Source: CAD feature listing. Evaluate the final solid. Frame: model axes, mm. Face numbers are marked on the shaded views. A direction names the side the tool comes from. Give positions to 0.01 mm unless a question says otherwise; leave off trailing zeros. Order: outer loops, then holes, each group sorted by start corner. A loop starts at its lowest first (then second) coordinate and runs counter-clockwise, first axis right, second up.
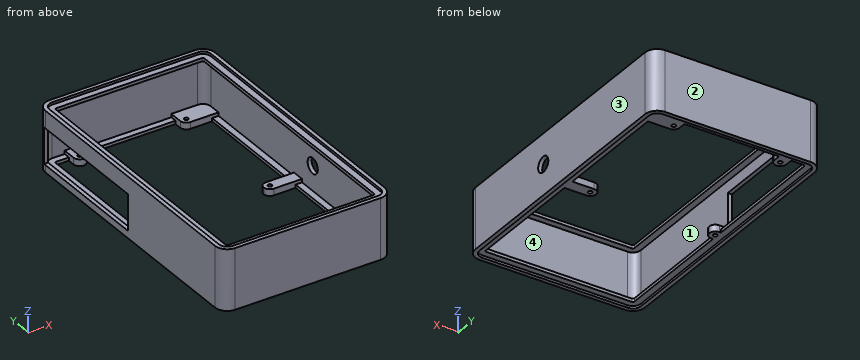
from build123d import *

# Parameters (mm, degrees)
SKETCH1_W               = 210
SKETCH1_H               = 350
SKETCH1_W_2             = 200
SKETCH1_H_2             = 340
BOSS_EXTRUDE1_DEPTH     = 75
FILLET1_R               = 15
FILLET2_R               = 10
BOSS_EXTRUDE2_START     = -4
BOSS_EXTRUDE2_DEPTH     = 4
CUT_EXTRUDE1_DEPTH      = 4
CUT_EXTRUDE1_DEPTH_BACK = 25
SKETCH3_W               = 44.5
SKETCH3_H               = 156.13
SKETCH3_H_2             = 2.62
SKETCH4_W               = 2
SKETCH4_H               = 2.62
CUT_EXTRUDE2_DEPTH      = 18
BOSS_EXTRUDE4_START     = -4
SKETCH5_R               = 2.55
BOSS_EXTRUDE4_DEPTH     = 8.23
SKETCH6_R               = 9.55
CUT_EXTRUDE4_DEPTH      = 22
CUT_EXTRUDE5_START      = -22
CUT_EXTRUDE5_DEPTH      = 22


with BuildPart() as part:
    # Sketch1 → Boss-Extrude1 (new body)
    with BuildSketch(Plane.XY):
        with Locations((105, 175)):
            Rectangle(SKETCH1_W, SKETCH1_H)
        with Locations((105, 175)):
            Rectangle(SKETCH1_W_2, SKETCH1_H_2, mode=Mode.SUBTRACT)
    extrude(amount=BOSS_EXTRUDE1_DEPTH)

    # Fillet1
    fillet1_edges = [part.edges().sort_by_distance(p)[0] for p in [
        (0, 350, 37.5),
        (210, 350, 37.5),
        (210, 0, 37.5),
        (0, 0, 37.5),
    ]]
    fillet(fillet1_edges, radius=FILLET1_R)

    # Fillet2
    fillet2_edges = [part.edges().sort_by_distance(p)[0] for p in [
        (5, 5, 37.5),
        (205, 5, 37.5),
        (205, 345, 37.5),
        (5, 345, 37.5),
    ]]
    fillet(fillet2_edges, radius=FILLET2_R)

    # Sketch2 → Boss-Extrude2 (add)
    with BuildSketch(Plane(origin=(0, 0, 3), x_dir=(-1, 0, 0), z_dir=(0, 0, -1)).offset(BOSS_EXTRUDE2_START)):
        with BuildLine():
            Line((-15, 5), (-195, 5))
            ThreePointArc((-195, 5), (-202.071067812, 7.928932188), (-205, 15))
            Line((-205, 15), (-205, 335))
            ThreePointArc((-205, 335), (-202.071067812, 342.071067812), (-195, 345))
            Line((-195, 345), (-15, 345))
            ThreePointArc((-15, 345), (-7.928932188, 342.071067812), (-5, 335))
            Line((-5, 335), (-5, 15))
            ThreePointArc((-5, 15), (-7.928932188, 7.928932188), (-15, 5))
        make_face()
        with BuildLine():
            Line((-13, 335), (-13, 15))
            ThreePointArc((-13, 15), (-13.585786438, 13.585786438), (-15, 13))
            Line((-15, 13), (-195, 13))
            ThreePointArc((-195, 13), (-196.414213562, 13.585786438), (-197, 15))
            Line((-197, 15), (-197, 335))
            ThreePointArc((-197, 335), (-196.414213562, 336.414213562), (-195, 337))
            Line((-195, 337), (-15, 337))
            ThreePointArc((-15, 337), (-13.585786438, 336.414213562), (-13, 335))
        make_face(mode=Mode.SUBTRACT)
    boss_extrude2 = extrude(amount=BOSS_EXTRUDE2_DEPTH)

    # Mirror1: Boss-Extrude2 across plane
    add(boss_extrude2.mirror(Plane(origin=(0, 0, 37.5), x_dir=(1, 0, 0), z_dir=(0, 0, -1))))

    # Sketch3 → Cut-Extrude1 (cut, two sides: drawn at the far end of the back side and taken through both)
    with BuildSketch(Plane(origin=(5, 0, 0), x_dir=(0, 0, -1), z_dir=(1, 0, 0)).offset(-CUT_EXTRUDE1_DEPTH_BACK)):
        with Locations((-31.25, 256.935)):
            Rectangle(SKETCH3_W, SKETCH3_H)
        with Locations((-31.25, 336.31)):
            Rectangle(SKETCH3_W, SKETCH3_H_2)
    extrude(amount=CUT_EXTRUDE1_DEPTH + CUT_EXTRUDE1_DEPTH_BACK, mode=Mode.SUBTRACT)

    # Sketch4 → Cut-Extrude2 (cut)
    with BuildSketch(Plane(origin=(5, 0, 0), x_dir=(0, 0, -1), z_dir=(1, 0, 0))):
        with Locations((-54.5, 336.31)):
            Rectangle(SKETCH4_W, SKETCH4_H)
        Polygon((-9, 337.62), (-53.5, 337.62), (-55.5, 337.62), (-55.5, 339.62), (-7, 339.62), (-7, 337.62), align=None)
        with Locations((-8, 336.31)):
            Rectangle(SKETCH4_W, SKETCH4_H)
    extrude(amount=CUT_EXTRUDE2_DEPTH, mode=Mode.SUBTRACT)

    # Sketch5 → Boss-Extrude4 (add)
    # profile 1 of 4: a face of its own
    with BuildSketch(Plane.XY.offset(7).offset(BOSS_EXTRUDE4_START)):
        with BuildLine():
            Line((15.06, 178.09), (5, 178.09))
            Line((5, 178.09), (5, 163.09))
            Line((5, 163.09), (15.06, 163.09))
            ThreePointArc((15.06, 163.09), (20.363300859, 165.286699141), (22.56, 170.59))
            ThreePointArc((22.56, 170.59), (20.363300859, 175.893300859), (15.06, 178.09))
        make_face()
        with Locations((15.06, 170.59)):
            Circle(SKETCH5_R, mode=Mode.SUBTRACT)
    # profile 2 of 4: a face of its own
    with BuildSketch(Plane.XY.offset(7).offset(BOSS_EXTRUDE4_START)):
        with BuildLine():
            Line((205, 163.09), (205, 178.09))
            Line((205, 178.09), (170, 178.09))
            ThreePointArc((170, 178.09), (164.696699141, 175.893300859), (162.5, 170.59))
            ThreePointArc((162.5, 170.59), (164.696699141, 165.286699141), (170, 163.09))
            Line((170, 163.09), (205, 163.09))
        make_face()
        with Locations((170, 170.59)):
            Circle(SKETCH5_R, mode=Mode.SUBTRACT)
    # profile 3 of 4: a face of its own
    with BuildSketch(Plane.XY.offset(7).offset(BOSS_EXTRUDE4_START)):
        with BuildLine():
            Line((195, 345), (162.5, 345))
            Line((162.5, 345), (162.5, 328.07))
            ThreePointArc((162.5, 328.07), (164.696699141, 322.766699141), (170, 320.57))
            Line((170, 320.57), (205, 320.57))
            Line((205, 320.57), (205, 335))
            ThreePointArc((205, 335), (202.071067812, 342.071067812), (195, 345))
        make_face()
        with Locations(Location((170, 328.07, 0), (0, 0, 180))):
            Circle(SKETCH5_R, mode=Mode.SUBTRACT)
    # profile 4 of 4: a face of its own
    with BuildSketch(Plane.XY.offset(7).offset(BOSS_EXTRUDE4_START)):
        with BuildLine():
            Line((45.42, 345), (30.42, 345))
            Line((30.42, 345), (30.42, 328.07))
            ThreePointArc((30.42, 328.07), (37.92, 320.57), (45.42, 328.07))
            Line((45.42, 328.07), (45.42, 345))
        make_face()
        with Locations((37.92, 328.07)):
            Circle(SKETCH5_R, mode=Mode.SUBTRACT)
    extrude(amount=BOSS_EXTRUDE4_DEPTH)

    # Sketch6 → Cut-Extrude4 (cut)
    with BuildSketch(Plane(origin=(210, 0, 0), x_dir=(0, 0, -1), z_dir=(1, 0, 0))):
        with Locations((-37.5, 143)):
            Circle(SKETCH6_R)
    extrude(amount=-CUT_EXTRUDE4_DEPTH, mode=Mode.SUBTRACT)

    # Sketch7 → Cut-Extrude5 (cut)
    with BuildSketch(Plane.XY.offset(11.23).offset(CUT_EXTRUDE5_START)):
        with BuildLine():
            Line((13, 169.087036261), (13, 172.092963739))
            ThreePointArc((13, 172.092963739), (12.51, 170.59), (13, 169.087036261))
        make_face()
    extrude(amount=CUT_EXTRUDE5_DEPTH, mode=Mode.SUBTRACT)


solid = part.part
(1) Section C-C, the plane y = 143. Return loops of the section in (x, z).
(2) Draft query along Z for the marked faces 1 and 2. Return one class per face: +Z half, -Z half, draft (parallel to the pull), parting line (faces both ways), or undercut.
(3) Section D-D, the plane x = 190.5. Return loops of the section in (y, z), plus the area to 3 significant figures.
(4) Line query: line 1 along X through (y, z) = (170.59, 6); line 2 along Y through (x, z) = (15.06, 5.5); line 3 along Y through (x, z) = (37.92, 7.25). Output: solid intervals per line, ascending.
(5) Section A-A, the plane y = 50.5. Return loops of the section in (x, z), plus the area to 3 significant figures.
(6) Section B-B, the plane x = 117. Return loops of the section in (y, z).
(7) Access query for the marked faces 3 and 4. Directions: +Z, -Z, +X, -X, +Y, -Y. A direction counts if a zero-diameter tool reaches every point of the face in a straight line with its end or side. Return the directions, or none.
(8) Pin query (flat end, axial travel): pin 1 Ø7.5 at (x, y) = (41, 329) entering from +Z; pin 2 Ø11.5 at (y, z) = (143, 37.5) entering from +X; pin 3 Ø1.4 at (x, z) = (3, 41.5) entering from -Y. Return the tip coordinate at first contact, or that it passes through.
Checks:
1. outline: (0, 0) - (5, 0) - (5, 3) - (13, 3) - (13, 7) - (5, 7) - (5, 68) - (13, 68) - (13, 72) - (5, 72) - (5, 75) - (0, 75) - close; (197, 3) - (205, 3) - (205, 0) - (210, 0) - (210, 27.95) - (205, 27.95) - (205, 7) - (197, 7) - close; (197, 68) - (205, 68) - (205, 47.05) - (210, 47.05) - (210, 75) - (205, 75) - (205, 72) - (197, 72) - close
2. face 1: undercut
2. face 2: draft
3. outline: (0, 0) - (5, 0) - (5, 3) - (13, 3) - (13, 7) - (5, 7) - (5, 68) - (13, 68) - (13, 72) - (5, 72) - (5, 75) - (0, 75) - close; (163.09, 3) - (178.09, 3) - (178.09, 11.23) - (163.09, 11.23) - close; (320.57, 3) - (345, 3) - (345, 0) - (350, 0) - (350, 75) - (345, 75) - (345, 72) - (337, 72) - (337, 68) - (345, 68) - (345, 11.23) - (320.57, 11.23) - close
3. area: 1,170 mm2
4. line 1: x = 0 to 12.51, 17.61 to 22.56, 162.5 to 167.45, 172.55 to 210
4. line 2: y = 0 to 13, 163.09 to 168.04, 173.14 to 178.09, 337 to 350
4. line 3: y = 0 to 5, 320.57 to 325.52, 330.62 to 350
5. outline: (0, 0) - (5, 0) - (5, 3) - (13, 3) - (13, 7) - (5, 7) - (5, 68) - (13, 68) - (13, 72) - (5, 72) - (5, 75) - (0, 75) - close; (197, 3) - (205, 3) - (205, 0) - (210, 0) - (210, 75) - (205, 75) - (205, 72) - (197, 72) - (197, 68) - (205, 68) - (205, 7) - (197, 7) - close
5. area: 878 mm2
6. outline: (0, 0) - (5, 0) - (5, 3) - (13, 3) - (13, 7) - (5, 7) - (5, 68) - (13, 68) - (13, 72) - (5, 72) - (5, 75) - (0, 75) - close; (337, 3) - (345, 3) - (345, 0) - (350, 0) - (350, 75) - (345, 75) - (345, 72) - (337, 72) - (337, 68) - (345, 68) - (345, 7) - (337, 7) - close
7. face 3: +Z, -Z, +X, +Y, -Y
7. face 4: none
8. pin 1: stops at z = 11.23
8. pin 2: stops at x = 5
8. pin 3: stops at y = 5.14
